from build123d import *

# Parameters (mm, degrees)
F1_DEPTH = 18
F3_R     = 2.5
F4_DEPTH = 10


with BuildPart() as f1:
    # F0 (on Front) → F1 (new body)
    with BuildSketch(Plane.XZ):
        with BuildLine():
            Line((0, -18.26), (0, 30))
            ThreePointArc((0, 30), (-3.356822, 28.705637), (-4.975665, 25.4927))
            Line((-4.975665, 25.4927), (-7.430809, 0.698745))
            ThreePointArc((-7.430809, 0.698745), (-7.450978, 0.002002), (-7.374057, -0.690776))
            Line((-7.374057, -0.690776), (-4.918914, -14.156821))
            ThreePointArc((-4.918914, -14.156821), (-3.202803, -17.099538), (0, -18.26))
        make_face()
    extrude(amount=F1_DEPTH)

    # F2: F1 across plane


with BuildPart() as f1_1:
    add(f1.part)
    add(f1.part.mirror(Plane.YZ))

    # F3 (on face) → F4 (join)
    with BuildSketch(Plane(origin=(0, 0, 0), x_dir=(-1, 0, 0), z_dir=(0, 1, 0))):
        Circle(F3_R)
    extrude(amount=F4_DEPTH)


solid = f1_1.part
Geometry check sheet. Reference: the model listing, model coordinates, mm. A direction names the side the tool comes from. Give positions to 0.01 mm unless a question says otherwise; leave off trailing zeros. Write each loop counter-clockwise with the first axis right and the second up, starting at its lowest first coordinate (ties: lowest second). Pieces come first, ordered by that corner, then holes.
1) Set-up check for faces 1 (the face through (0.54, 4.93, -2.44)), 2 (the face through (-6.164, -8.874, -7.33)): record each of +Z, -Z, +X, -X, +Y, -Y from which the full face is reachable in a straight line by a thin tool's end or side.
Values follow:
face 1: +Y
face 2: -Z, -X, +Y, -Y
2) Cross-section at C-C (x = -3.75). Record the boundary of the cut face in (y, z), plus the area to 3 significant figures.
Values follow:
outline: (-18, -16.57) - (0, -16.57) - (0, 28.31) - (-18, 28.31) - close
area: 808 mm2
3) Go/stop test with flat-tipped pins: pin 1 Ø8 at (y, z) = (-7, 17.5) entering from +X; pin 2 Ø3 at (x, y) = (1.5, -11.5) entering from -Z; pin 3 Ø2 at (x, y) = (3.5, -10) entering from -Z; pin 4 Ø1 at (x, y) = (2.5, -8.5) entering from +Z. Record where each tip stops, or that it passes through.
Values follow:
pin 1: stops at x = 6.16
pin 2: stops at z = -18.26
pin 3: stops at z = -17.59
pin 4: stops at z = 29.58
4) Cross-section at B-B (z = 2). Record the boundary of the cut face in (x, y).
Values follow:
outline: (-7.3, -18) - (7.3, -18) - (7.3, 0) - (1.5, 0) - (1.5, 10) - (-1.5, 10) - (-1.5, 0) - (-7.3, 0) - close
5) Cross-section at A-A (y = -7.5). Record the boundary of the cut face in (x, z).
Values follow:
outline: (-7.43, 0.7) arc R5 ccw to (-7.37, -0.69) - (-4.92, -14.16) arc R5 ccw to (4.92, -14.16) - (7.37, -0.69) arc R5 ccw to (7.43, 0.7) - (4.98, 25.49) arc R5 ccw to (-4.98, 25.49) - close
6) Cross-section at D-D (y = 5.75). Record the boundary of the cut face in (x, z).
Values follow:
outline: circle Ø5 at (0, 0)
7) Thickness scan on line 1 (Y direction, x = -5, z = -13); line 2 (X direction, y = -11.75, z = -13); line 3 (Z direction, x = -2.25, y = 6). Record the ranges inside material, lowest first.
Values follow:
line 1: y = -18 to 0
line 2: x = -5.13 to 5.13
line 3: z = -1.09 to 1.09
